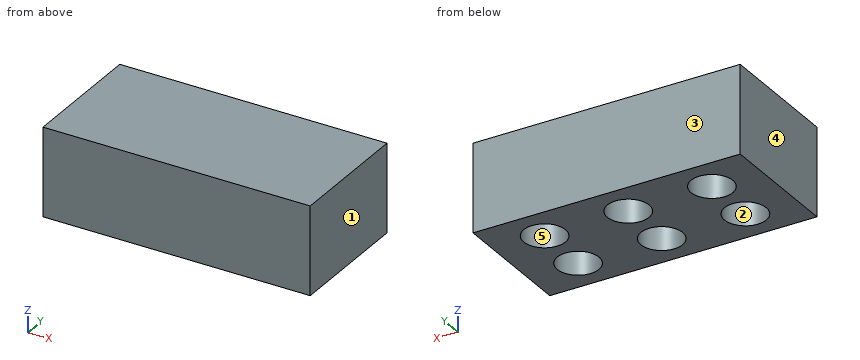
from build123d import *

# Parameters (mm, degrees)
CYLINDER001_R     = 18
CYLINDER001_DEPTH = 76
CYLINDER002_R     = 18
CYLINDER002_DEPTH = 76
CYLINDER003_R     = 18
CYLINDER003_DEPTH = 76
CYLINDER004_R     = 18
CYLINDER004_DEPTH = 76
CYLINDER005_R     = 18
CYLINDER005_DEPTH = 76
CYLINDER_R        = 18
CYLINDER_DEPTH    = 76
BOX_W             = 230
BOX_H             = 110
BOX_DEPTH         = 76


with BuildPart() as cylinder001:
    # Cylinder001 → Cylinder001 (new body)
    with BuildSketch(Plane(origin=(115, 31, 0), x_dir=(1, 0, 0), z_dir=(0, 0, 1))):
        Circle(CYLINDER001_R)
    extrude(amount=CYLINDER001_DEPTH)


with BuildPart() as cylinder002:
    # Cylinder002 → Cylinder002 (new body)
    with BuildSketch(Plane(origin=(187, 31, 0), x_dir=(1, 0, 0), z_dir=(0, 0, 1))):
        Circle(CYLINDER002_R)
    extrude(amount=CYLINDER002_DEPTH)


with BuildPart() as cylinder003:
    # Cylinder003 → Cylinder003 (new body)
    with BuildSketch(Plane(origin=(187, 79, 0), x_dir=(1, 0, 0), z_dir=(0, 0, 1))):
        Circle(CYLINDER003_R)
    extrude(amount=CYLINDER003_DEPTH)


with BuildPart() as cylinder004:
    # Cylinder004 → Cylinder004 (new body)
    with BuildSketch(Plane(origin=(115, 79, 0), x_dir=(1, 0, 0), z_dir=(0, 0, 1))):
        Circle(CYLINDER004_R)
    extrude(amount=CYLINDER004_DEPTH)


with BuildPart() as cylinder005:
    # Cylinder005 → Cylinder005 (new body)
    with BuildSketch(Plane(origin=(43, 79, 0), x_dir=(1, 0, 0), z_dir=(0, 0, 1))):
        Circle(CYLINDER005_R)
    extrude(amount=CYLINDER005_DEPTH)


with BuildPart() as obj1:
    # Cylinder → Cylinder (new body)
    with BuildSketch(Plane(origin=(43, 31, 0), x_dir=(1, 0, 0), z_dir=(0, 0, 1))):
        Circle(CYLINDER_R)
    extrude(amount=CYLINDER_DEPTH)

    # Fusion: union Cylinder001, Cylinder002, Cylinder003, Cylinder004, Cylinder005
    add(cylinder001.part)
    add(cylinder002.part)
    add(cylinder003.part)
    add(cylinder004.part)
    add(cylinder005.part)


with BuildPart() as obj2:
    # Box → Box (new body)
    with BuildSketch(Plane.XY.offset(1)):
        with Locations((115, 55)):
            Rectangle(BOX_W, BOX_H)
    extrude(amount=BOX_DEPTH)

    # Cut: cut obj1
    add(obj1.part, mode=Mode.SUBTRACT)


solid = obj2.part
The model under review builds one solid part; all positions refer to its coordinate system, in mm. Face numbers are marked on the shaded views. A direction names the side the tool comes from. Give positions to 0.01 mm unless a question says otherwise; leave off trailing zeros. Loops run counter-clockwise (first coordinate to the right, second up) from the corner with the lowest first, then second, coordinate; pieces in that order, holes last. Notation, with made-up numbers: (11.25, -6.75) -> (50.25, -6.75) arc R23 ccw to (50.25, 13.25) -> close; hole circle Ø3 at (77, 52). An arc over 180 degrees is marked (long way). Put each result on its own line as item: value. Start each with the question number.
1. Clearance check with a flat-ended pin moving along its axis: P1, Ø10, axis at x = 107.5, y = 78.5, coming from the -Z side. State where the tip first meets the part, or that it passes through.
2. For the marked faces 4 and 5, list the 3-axis set-ups (+Z, -Z, +X, -X, +Y, -Y) from which the entire face can be reached by the end or side of a thin tool; tool diameter is ignored.
3. We need section D-D on y = 21. State the section outline as (x, z) points.
4. Mouldability with a two-part tool opening along Y and no side actions: class the marked faces 1, 2 and 3 as released by +Y, released by -Y, zero draft, split by the parting line, or undercut.
5. Wall thickness on probe 1 along Y at (x, z) = (115, 38); probe 2 along X at (y, z) = (30.5, 44.5); probe 3 along X at (y, z) = (73.5, 59.5): over which ranges is each line inside the solid? List them lowest first.
6. We need section A-A on y = 79. State the section outline as (x, z) points.
7. We need section C-C on x = 43. State the section outline as (y, z) points.
8. We need section B-B on z = 53.5. State the section outline as (x, y) points.
Determined:
1. P1: z = 76
2. face 4: +Z, -Z, -X, +Y, -Y
2. face 5: -Z
3. outline: (0, 1) -> (28.03, 1) -> (28.03, 76) -> (57.97, 76) -> (57.97, 1) -> (100.03, 1) -> (100.03, 76) -> (129.97, 76) -> (129.97, 1) -> (172.03, 1) -> (172.03, 76) -> (201.97, 76) -> (201.97, 1) -> (230, 1) -> (230, 77) -> (0, 77) -> close
4. face 1: zero draft
4. face 2: undercut
4. face 3: released by +Y
5. probe 1: 0 to 13, 49 to 61, 97 to 110
5. probe 2: 0 to 25.01, 60.99 to 97.01, 132.99 to 169.01, 204.99 to 230
5. probe 3: 0 to 25.86, 60.14 to 97.86, 132.14 to 169.86, 204.14 to 230
6. outline: (0, 1) -> (25, 1) -> (25, 76) -> (61, 76) -> (61, 1) -> (97, 1) -> (97, 76) -> (133, 76) -> (133, 1) -> (169, 1) -> (169, 76) -> (205, 76) -> (205, 1) -> (230, 1) -> (230, 77) -> (0, 77) -> close
7. outline: (0, 1) -> (13, 1) -> (13, 76) -> (49, 76) -> (49, 1) -> (61, 1) -> (61, 76) -> (97, 76) -> (97, 1) -> (110, 1) -> (110, 77) -> (0, 77) -> close
8. outline: (0, 0) -> (230, 0) -> (230, 110) -> (0, 110) -> close; hole circle Ø36 at (43, 31); hole circle Ø36 at (43, 79); hole circle Ø36 at (115, 31); hole circle Ø36 at (115, 79); hole circle Ø36 at (187, 31); hole circle Ø36 at (187, 79)
